Autodesk Fusion 360 part; units mm, degrees
sketch "Sketch1" plane through (0, 0, 0) normal (0, 0, 1) x (1, 0, 0)
  line L0 (0, 0) -> (-25, 0) construction
  line L1 (-25, 0) -> (-25, 17)
  line L2 (-22, 20) -> (0, 20)
  line L3 (0, 20) -> (0, 0) construction
  circle A0 centre (-12, 9) radius 2
  arc A1 (-22, 20) -> (-25, 17) centre (-22, 17) ccw
  circle A2 centre (-12, -9) radius 2
  arc A3 (-25, -17) -> (-22, -20) centre (-22, -17) ccw
  line L4 (-22, -20) -> (0, -20)
  line L5 (-25, 0) -> (-25, -17)
  arc A4 (25, 17) -> (22, 20) centre (22, 17) ccw
  arc A5 (22, -20) -> (25, -17) centre (22, -17) ccw
  line L6 (22, -20) -> (0, -20)
  line L7 (22, 20) -> (0, 20)
  line L8 (25, 0) -> (25, 17)
  circle A6 centre (12, -9) radius 2
  circle A7 centre (12, 9) radius 2
  line L9 (25, 0) -> (25, -17)
  point P0 (-25, 20)
  point P1 (-25, -20)
  point P2 (25, 20)
  point P3 (25, -20)
  dimension "d1" = 20
  dimension "d2" = 25
  dimension "d3" = 12
  dimension "d4" = 9
  dimension "d5" = 4
  dimension "d6" = 3
extrude "Extrude1" add sketch "Sketch1" along normal blind 3
Input: part model. Units: mm. Frame: model coordinates. Give positions to 0.01 mm unless a question says otherwise; leave off trailing zeros. Loops run counter-clockwise (first coordinate to the right, second up) from the corner with the lowest first, then second, coordinate; pieces in that order, holes last.
1) Mould query, pull axis X, two halves, no side actions, for faces 1 (the flat face through (0, 0, 3)), 2 (the cylindrical face through (24.1, 19.14, 1.48)), 3 (the cylindrical face through (-13.474, -10.352, 1.479)). Classes: released by +X, released by -X, zero draft, split by the parting line, or undercut.
A:
face 1: zero draft
face 2: released by +X
face 3: undercut
2) Section query B-B on y = 9. Return the cut outline in (x, z), and give its area (3 significant figures).
A:
outline: (-25, 0) - (-14, 0) - (-14, 3) - (-25, 3) - close; (-10, 0) - (10, 0) - (10, 3) - (-10, 3) - close; (14, 0) - (25, 0) - (25, 3) - (14, 3) - close
area: 126 mm2
3) Section query A-A on z = 2.3. Return the cut outline in (x, y), and give its area (3 significant figures).
A:
outline: (-25, -17) arc R3 ccw to (-22, -20) - (22, -20) arc R3 ccw to (25, -17) - (25, 17) arc R3 ccw to (22, 20) - (-22, 20) arc R3 ccw to (-25, 17) - close; hole circle Ø4 at (-12, -9); hole circle Ø4 at (-12, 9); hole circle Ø4 at (12, -9); hole circle Ø4 at (12, 9)
area: 1,940 mm2
4) Line query: L1, parallel to Y at x = -12, z = 0.7; L2, parallel to X at y = 10, z = 1.4; L3, parallel to X at y = 9.5, z = 1.3. Output: solid intervals per line, ascending.
A:
L1: y = -20 to -11, -7 to 7, 11 to 20
L2: x = -25 to -13.73, -10.27 to 10.27, 13.73 to 25
L3: x = -25 to -13.94, -10.06 to 10.06, 13.94 to 25
5) Section query C-C on x = 12. Return the cut outline in (y, z), and give its area (3 significant figures).
A:
outline: (-20, 0) - (-11, 0) - (-11, 3) - (-20, 3) - close; (-7, 0) - (7, 0) - (7, 3) - (-7, 3) - close; (11, 0) - (20, 0) - (20, 3) - (11, 3) - close
area: 96.0 mm2
